Read the model definition and answer for the solid it produces. Units are mm, in the model's axes. Face numbers are marked on the shaded views. A direction names the side the tool comes from. Give positions to 0.01 mm unless a question says otherwise; leave off trailing zeros. Loops run counter-clockwise (first coordinate to the right, second up) from the corner with the lowest first, then second, coordinate; pieces in that order, holes last. Notation, with made-up numbers: (5.5, 48) -> (29.5, 48) arc R31 cw to (29.5, 76) -> close; hole circle Ø9 at (49, -28). An arc over 180 degrees is marked (long way). One line per item, written item: value. Start each with the question number.
from build123d import *

# Parameters (mm, degrees)
SKETCH_1_W          = 40
SKETCH_1_H          = 40
EXTRUDE_1_DEPTH     = 21
SKETCH_2_W          = 14.5
SKETCH_2_H          = 37
CUT_EXTRUDE_1_DEPTH = 61.340699366
CUT_EXTRUDE_2_REACH = 62.341
SKETCH_3_W          = 24.017804412
SKETCH_3_H          = 26
SKETCH_4_W          = 40
SKETCH_4_H          = 8
CUT_EXTRUDE_3_DEPTH = 16
SKETCH_5_W          = 40
SKETCH_5_H          = 13
EXTRUDE_3_DEPTH     = 40
SKETCH_6_W          = 40
SKETCH_6_H          = 13
EXTRUDE_4_DEPTH     = 50
FILLET_1_R          = 20
FILLET_2_R          = 20
CUT_EXTRUDE_4_REACH = 90.436
SKETCH_7_R          = 2


with BuildPart() as part:
    # 草图1 → 凸台-拉伸1 (new body)
    with BuildSketch(Plane.XY):
        with Locations((20, 20)):
            Rectangle(SKETCH_1_W, SKETCH_1_H)
    extrude(amount=EXTRUDE_1_DEPTH)

    # 草图2 → 切除-拉伸1 (cut, through all)
    with BuildSketch(Plane(origin=(40, 0, 0), x_dir=(0, 0, -1), z_dir=(1, 0, 0))):
        with Locations((-10.75, 21.5)):
            Rectangle(SKETCH_2_W, SKETCH_2_H)
    extrude(amount=-CUT_EXTRUDE_1_DEPTH, mode=Mode.SUBTRACT)

    # 草图3 → 切除-拉伸2 (cut, up to next)
    with BuildSketch(Plane.XY.offset(21), mode=Mode.PRIVATE) as cut_extrude_2_sk1:
        with Locations((19.991097794, 27)):
            Rectangle(SKETCH_3_W, SKETCH_3_H)
    cut_extrude_2_tool1 = extrude(cut_extrude_2_sk1.sketch, amount=-CUT_EXTRUDE_2_REACH, mode=Mode.PRIVATE) & part.part
    add(cut_extrude_2_tool1.solids().sort_by_distance((19.991098, 27, 21))[0], mode=Mode.SUBTRACT)

    # 草图4 → 切除-拉伸3 (cut)
    with BuildSketch(Plane(origin=(0, 0, 0), x_dir=(-1, 0, 0), z_dir=(0, 0, -1))):
        with Locations((-20, 36)):
            Rectangle(SKETCH_4_W, SKETCH_4_H)
    extrude(amount=-CUT_EXTRUDE_3_DEPTH, mode=Mode.SUBTRACT)

    # 草图5 → 凸台-拉伸3 (add)
    with BuildSketch(Plane(origin=(0, 0, 0), x_dir=(-1, 0, 0), z_dir=(0, 0, -1))):
        with Locations((-20, 6.5)):
            Rectangle(SKETCH_5_W, SKETCH_5_H)
    extrude(amount=EXTRUDE_3_DEPTH)

    # 草图6 → 凸台-拉伸4 (add)
    with BuildSketch(Plane.XZ):
        with Locations((20, -33.5)):
            Rectangle(SKETCH_6_W, SKETCH_6_H)
    extrude(amount=EXTRUDE_4_DEPTH)

    # 圆角1
    fillet_1_edges = [part.edges().sort_by_distance(p)[0] for p in [
        (20, 0, -27),
    ]]
    fillet(fillet_1_edges, radius=FILLET_1_R)

    # 圆角2
    fillet_2_edges = [part.edges().sort_by_distance(p)[0] for p in [
        (20, 13, -40),
    ]]
    fillet(fillet_2_edges, radius=FILLET_2_R)

    # 草图7 → 切除-拉伸4 (cut, up to next)
    with BuildSketch(Plane(origin=(0, 0, -40), x_dir=(-1, 0, 0), z_dir=(0, 0, -1)), mode=Mode.PRIVATE) as cut_extrude_4_sk1:
        with Locations((-31, -44)):
            Circle(SKETCH_7_R)
    cut_extrude_4_tool1 = extrude(cut_extrude_4_sk1.sketch, amount=-CUT_EXTRUDE_4_REACH, mode=Mode.PRIVATE) & part.part
    # 草图7 → 切除-拉伸4 (cut, up to next)
    with BuildSketch(Plane(origin=(0, 0, -40), x_dir=(-1, 0, 0), z_dir=(0, 0, -1)), mode=Mode.PRIVATE) as cut_extrude_4_sk2:
        with Locations((-9, -44)):
            Circle(SKETCH_7_R)
    cut_extrude_4_tool2 = extrude(cut_extrude_4_sk2.sketch, amount=-CUT_EXTRUDE_4_REACH, mode=Mode.PRIVATE) & part.part
    add(cut_extrude_4_tool1.solids().sort_by_distance((31, -44, -40))[0], mode=Mode.SUBTRACT)
    add(cut_extrude_4_tool2.solids().sort_by_distance((9, -44, -40))[0], mode=Mode.SUBTRACT)


solid = part.part
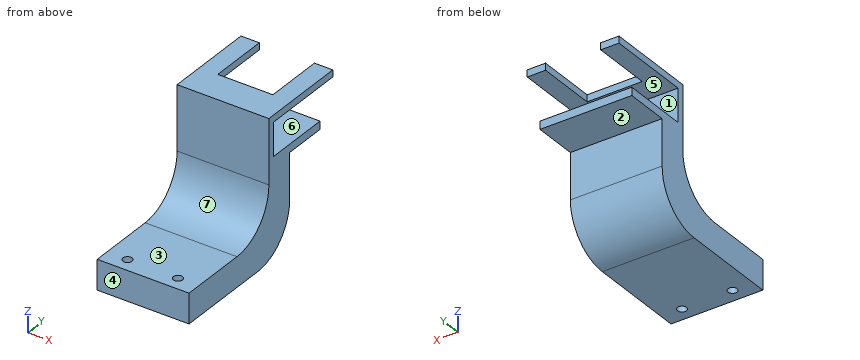
Item 1: Flat-ended cylindrical pins translate along their axes: pin 1 (5 mm diameter, centred on x = 6.5, z = 9.5, fed in from +Y); pin 2 (6.5 mm diameter, centred on x = 31, y = -44, fed in from +Z); pin 3 (5.5 mm diameter, centred on x = 18.5, y = 23.5, fed in from -Z). Find the tip coordinate at first contact, or state that the pin passes through.
Item 2: Section C-C, the plane x = 34.5 is taken. Determine the outline of the cut face in (y, z), plus the area to 3 significant figures.
Item 3: Section B-B, the plane y = -44 is taken. Determine the outline of the cut face in (x, z), plus the area to 3 significant figures.
Item 4: Determine the mould class of the marked faces 4, 5, 6 and 7 for opening direction Z: pulls with the +Z half, pulls with the -Z half, needs draft (parallel to the pull), parting line crosses it, or undercut.
Item 5: For the marked faces 1, 2 and 3, determine the directions among +Z, -Z, +X, -X, +Y, -Y from which every point of the face is accessible in a straight line to the end or side of a thin tool.
Item 6: Section D-D, the plane z = -6 is taken. Determine the outline of the cut face in (x, y).
Item 7: Section A-A, the plane x = 9 is taken. Determine the outline of the cut face in (y, z).
Item 8: Consider L1, parallel to Z at x = 11.5, y = 21; L2, parallel to Y at x = 26, z = -7.5; L3, parallel to Z at x = 13, y = 10.5. Determine where each line is inside the solid, lowest interval first. Write a range as [from, to].
Computed values:
1. pin 1: y = 3
1. pin 2: z = -27
1. pin 3: z = 0
2. outline: (-50, -40) -> (-7, -40) arc R20 ccw to (13, -20) -> (13, 0) -> (32, 0) -> (32, 3.5) -> (3, 3.5) -> (3, 18) -> (40, 18) -> (40, 21) -> (0, 21) -> (0, -7) arc R20 cw to (-20, -27) -> (-50, -27) -> close
2. area: 1,450 mm²
3. outline: (0, -40) -> (7, -40) -> (7, -27) -> (0, -27) -> close; (11, -40) -> (29, -40) -> (29, -27) -> (11, -27) -> close; (33, -40) -> (40, -40) -> (40, -27) -> (33, -27) -> close
3. area: 416 mm²
4. face 4: needs draft
4. face 5: undercut
4. face 6: undercut
4. face 7: pulls with the +Z half
5. face 1: +X, -X, +Y
5. face 2: -Z, +X, -X, +Y
5. face 3: +Z, +X, -X, -Y
6. outline: (0, 0) -> (40, 0) -> (40, 13) -> (0, 13) -> close
7. outline: (-50, -40) -> (-46, -40) -> (-46, -27) -> (-50, -27) -> close; (-42, -40) -> (-7, -40) arc R20 ccw to (13, -20) -> (13, 0) -> (32, 0) -> (32, 3.5) -> (3, 3.5) -> (3, 18) -> (14, 18) -> (14, 21) -> (0, 21) -> (0, -7) arc R20 cw to (-20, -27) -> (-42, -27) -> close
8. L1: [0, 3.5]
8. L2: [-0.01, 13]
8. L3: [-29.68, 3.5], [18, 21]
